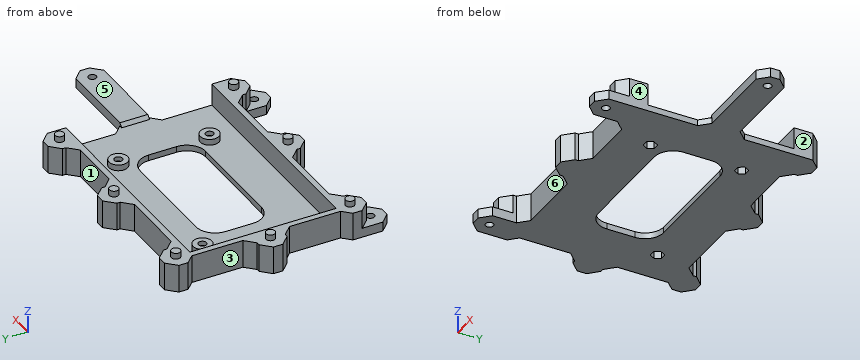
from build123d import *

# Parameters (mm, degrees)
F0_W          = 121.6
F0_H          = 78.3
F0_R          = 2.125
F1_DEPTH      = 3.2
F2_R          = 5
F2_R_2        = 2.125
F3_DEPTH      = 3.2
F5_DEPTH      = 4
F7_DEPTH      = 15
F8_R          = 2.425
F9_DEPTH      = 3.2
F11_W         = 15
F11_H         = 17.8
F11_R         = 2.125
F12_DEPTH     = 5
F13_T1_DEPTH  = 3.2
F13_T3_DEPTH  = 15
F13_T5_DEPTH  = 30.7168298797
F13_T7_DEPTH  = 22.8584149398
F13_T9_DEPTH  = 40.7168298797
F13_T14_DEPTH = 14.6584149398
F13_T19_DEPTH = 14.6584149398
F13_T24_DEPTH = 40.7168298797
F13_T29_DEPTH = 40.7168298797
F13_T34_DEPTH = 40.7168298797


# Not quite as in the source:
# - a fillet or chamfer that OpenCascade refuses, or shapes differently, is made with other operations: its cross-section is extruded or revolved along the edge and cut away or added
# - two fillets or chamfers of one size are made in one step
# - a feature of the source that left no trace in its solid (it failed there, or was rolled back) is left out
# - a feature names something its author has since deleted; it is built from what else it names


with BuildPart() as f1:
    # F0 (on Top) → F1 (new body)
    with BuildSketch(Plane.XY):
        Rectangle(F0_W, F0_H)
        with Locations((35.5, -24.05)):
            Circle(F0_R, mode=Mode.SUBTRACT)
        with BuildLine():
            ThreePointArc((37.5, -7.5), (34.5710678119, -14.5710678119), (27.5, -17.5))
            Line((27.5, -17.5), (-27.5, -17.5))
            ThreePointArc((-27.5, -17.5), (-34.5710678119, -14.5710678119), (-37.5, -7.5))
            Line((-37.5, -7.5), (-37.5, 7.5))
            ThreePointArc((-37.5, 7.5), (-34.5710678119, 14.5710678119), (-27.5, 17.5))
            Line((-27.5, 17.5), (27.5, 17.5))
            ThreePointArc((27.5, 17.5), (34.5710678119, 14.5710678119), (37.5, 7.5))
            Line((37.5, 7.5), (37.5, -7.5))
        make_face(mode=Mode.SUBTRACT)
        with Locations((-45.72, 24.15)):
            Circle(F0_R, mode=Mode.SUBTRACT)
        with Locations((36.8, 24.15)):
            Circle(F0_R, mode=Mode.SUBTRACT)
    extrude(amount=F1_DEPTH)

    # F2 (on face) → F3 (join)
    with BuildSketch(Plane.XY.offset(3.2)):
        with Locations((-45.72, 24.15)):
            Circle(F2_R)
        with Locations((-45.72, 24.15)):
            Circle(F2_R_2, mode=Mode.SUBTRACT)
        with Locations((36.8, 24.15)):
            Circle(F2_R)
        with Locations((36.8, 24.15)):
            Circle(F2_R_2, mode=Mode.SUBTRACT)
        with Locations((35.5, -24.05)):
            Circle(F2_R)
        with Locations((35.5, -24.05)):
            Circle(F2_R_2, mode=Mode.SUBTRACT)
    extrude(amount=F3_DEPTH)

    # F4 (on face) → F5 (cut)
    with BuildSketch(Plane(origin=(0, 0, 0), x_dir=(1, 0, 0), z_dir=(0, 0, -1))):
        Polygon((-44.0312504626, -21.225), (-47.4087495374, -21.225), (-49.0974990748, -24.15), (-47.4087495374, -27.075), (-44.0312504626, -27.075), (-42.3425009252, -24.15), align=None)
        Polygon((38.4887495374, -21.225), (35.1112504626, -21.225), (33.4225009252, -24.15), (35.1112504626, -27.075), (38.4887495374, -27.075), (40.1774990748, -24.15), align=None)
        Polygon((33.8112504626, 21.125), (37.1887495374, 21.125), (38.8774990748, 24.05), (37.1887495374, 26.975), (33.8112504626, 26.975), (32.1225009252, 24.05), align=None)
    extrude(amount=-F5_DEPTH, mode=Mode.SUBTRACT)

    # F6 (on Top) → F7 (join)
    with BuildSketch(Plane.XY):
        Polygon((-60.8, 39.15), (60.8, 39.15), (60.8, 54.15), (45.8, 54.15), (45.8, 42.35), (7.5, 42.35), (7.5, 54.15), (-7.5, 54.15), (-7.5, 42.35), (-53.3, 42.35), (-53.3, 54.15), (-68.3, 54.15), (-68.3, 39.15), (-64, 39.15), (-64, 7.5), (-75.8, 7.5), (-75.8, -7.5), (-64, -7.5), (-64, -39.15), (-68.3, -39.15), (-68.3, -54.15), (-53.3, -54.15), (-53.3, -42.35), (-7.5, -42.35), (-7.5, -54.15), (7.5, -54.15), (7.5, -42.35), (45.8, -42.35), (45.8, -54.15), (60.8, -54.15), (60.8, -39.15), (-60.8, -39.15), align=None)
    extrude(amount=F7_DEPTH)

    # F8 (on face) → F9 (join)
    with BuildSketch(Plane.XY.offset(15)):
        with Locations((53.3, 46.65)):
            Circle(F8_R)
        with Locations((0, 46.65)):
            Circle(F8_R)
        with Locations((-60.8, 46.65)):
            Circle(F8_R)
        with Locations((-68.3, 0)):
            Circle(F8_R)
        with Locations((-60.8, -46.65)):
            Circle(F8_R)
        with Locations((0, -46.65)):
            Circle(F8_R)
        with Locations((53.3, -46.65)):
            Circle(F8_R)
    extrude(amount=F9_DEPTH)

    # F11 (on Top) → F12 (join)
    with BuildSketch(Plane.XY):
        with Locations((53.3, -56.25)):
            Rectangle(F11_W, F11_H)
        with Locations((53.3, -57.65)):
            Circle(F11_R, mode=Mode.SUBTRACT)
        with Locations((-60.8, -56.25)):
            Rectangle(F11_W, F11_H)
        with Locations((-60.8, -57.65)):
            Circle(F11_R, mode=Mode.SUBTRACT)
        Polygon((60.8, -7.5), (64, -7.5), (114, -7.5), (114, 7.5), (64, 7.5), (60.8, 7.5), align=None)
        with Locations((106.5, 0)):
            Circle(F11_R, mode=Mode.SUBTRACT)
    extrude(amount=F12_DEPTH)

    # F13: chamfer of 5 on 37 edges, made by hand

    # F13_s2 → F13_t1 (join)
    with BuildSketch(Plane.XY):
        Polygon((65.8, 7.5), (60.8, 12.5), (60.8, 7.5), align=None)
        Polygon((60.8, -12.5), (65.8, -7.5), (60.8, -7.5), align=None)
    extrude(amount=F13_T1_DEPTH)

    # F13_s4 → F13_t3 (join)
    with BuildSketch(Plane.XY):
        Polygon((45.8, 47.35), (40.8, 42.35), (45.8, 42.35), align=None)
        Polygon((12.5, 42.35), (7.5, 47.35), (7.5, 42.35), align=None)
        Polygon((-7.5, 47.35), (-12.5, 42.35), (-7.5, 42.35), align=None)
        Polygon((-48.3, 42.35), (-53.3, 47.35), (-53.3, 42.35), align=None)
        Polygon((-64, 12.5), (-69, 7.5), (-64, 7.5), align=None)
        Polygon((-69, -7.5), (-64, -12.5), (-64, -7.5), align=None)
        Polygon((-53.3, -47.35), (-48.3, -42.35), (-53.3, -42.35), align=None)
        Polygon((-12.5, -42.35), (-7.5, -47.35), (-7.5, -42.35), align=None)
        Polygon((7.5, -47.35), (12.5, -42.35), (7.5, -42.35), align=None)
        Polygon((40.8, -42.35), (45.8, -47.35), (45.8, -42.35), align=None)
    extrude(amount=F13_T3_DEPTH)

    # F13_s6 → F13_t5 (cut)
    with BuildSketch(Plane.XY.offset(-12.8584149398)):
        Polygon((-68.3, -60.15), (-63.3, -65.15), (-68.3, -65.15), align=None)
        Polygon((-58.3, -65.15), (-53.3, -60.15), (-53.3, -65.15), align=None)
        Polygon((50.8, -65.15), (45.8, -60.15), (45.8, -65.15), align=None)
        Polygon((60.8, -60.15), (55.8, -65.15), (60.8, -65.15), align=None)
        Polygon((114, 2.5), (109, 7.5), (114, 7.5), align=None)
        Polygon((109, -7.5), (114, -2.5), (114, -7.5), align=None)
    extrude(amount=F13_T5_DEPTH, mode=Mode.SUBTRACT)

    # F13_s8 → F13_t7 (cut)
    with BuildSketch(Plane.XY.offset(5)):
        Polygon((60.8, -49.15), (55.8, -54.15), (60.8, -54.15), align=None)
        Polygon((-68.3, -49.15), (-63.3, -54.15), (-68.3, -54.15), align=None)
        Polygon((-53.3, -49.15), (-58.3, -54.15), (-53.3, -54.15), align=None)
        Polygon((50.8, -54.15), (45.8, -49.15), (45.8, -54.15), align=None)
    extrude(amount=F13_T7_DEPTH, mode=Mode.SUBTRACT)

    # F13_s10 → F13_t9 (cut)
    with BuildSketch(Plane.XY.offset(-12.8584149398)):
        Polygon((60.8, 49.15), (55.8, 54.15), (60.8, 54.15), align=None)
        Polygon((50.8, 54.15), (45.8, 49.15), (45.8, 54.15), align=None)
        Polygon((7.5, 49.15), (2.5, 54.15), (7.5, 54.15), align=None)
        Polygon((-2.5, 54.15), (-7.5, 49.15), (-7.5, 54.15), align=None)
        Polygon((-53.3, 49.15), (-58.3, 54.15), (-53.3, 54.15), align=None)
        Polygon((-63.3, 54.15), (-68.3, 49.15), (-68.3, 54.15), align=None)
        Polygon((-70.8, 7.5), (-75.8, 2.5), (-75.8, 7.5), align=None)
        Polygon((-75.8, -2.5), (-70.8, -7.5), (-75.8, -7.5), align=None)
        Polygon((-7.5, -49.15), (-2.5, -54.15), (-7.5, -54.15), align=None)
        Polygon((2.5, -54.15), (7.5, -49.15), (7.5, -54.15), align=None)
    extrude(amount=F13_T9_DEPTH, mode=Mode.SUBTRACT)


with BuildPart() as f13_tool12:
    # F13_s13 → F13_t14 (new body)
    with BuildSketch(Plane.XY.offset(3.2)):
        Polygon((65.8, 7.5), (60.8, 2.5), (60.8, 7.5), align=None)
    extrude(amount=F13_T14_DEPTH)

    split(bisect_by=Plane(origin=(30.4, 0, -30.4), x_dir=(0, 1, 0), z_dir=(-0.7071067812, 0, 0.7071067812)), keep=Keep.TOP)


with BuildPart() as f1_1:
    add(f1.part)

    # F13_t11: cut F13_tool12
    add(f13_tool12.part, mode=Mode.SUBTRACT)


with BuildPart() as f13_tool17:
    # F13_s18 → F13_t19 (new body)
    with BuildSketch(Plane.XY.offset(3.2)):
        Polygon((65.8, -7.5), (60.8, -2.5), (60.8, -7.5), align=None)
    extrude(amount=F13_T19_DEPTH)

    split(bisect_by=Plane(origin=(30.4, 0, -30.4), x_dir=(0, 1, 0), z_dir=(-0.7071067812, 0, 0.7071067812)), keep=Keep.TOP)


with BuildPart() as f1_2:
    add(f1_1.part)

    # F13_t16: cut F13_tool17
    add(f13_tool17.part, mode=Mode.SUBTRACT)


with BuildPart() as f13_tool22:
    # F13_s23 → F13_t24 (new body)
    with BuildSketch(Plane.XZ.offset(-20.3584149398)):
        Polygon((60.8, 0), (65.8, 5), (60.8, 5), align=None)
    extrude(amount=F13_T24_DEPTH)

    split(bisect_by=Plane.XY.offset(3.2), keep=Keep.TOP)


with BuildPart() as f1_3:
    add(f1_2.part)

    # F13_t21: cut F13_tool22
    add(f13_tool22.part, mode=Mode.SUBTRACT)


with BuildPart() as f13_tool27:
    # F13_s28 → F13_t29 (new body)
    with BuildSketch(Plane.XY.offset(-12.8584149398)):
        Polygon((-68.3, 44.15), (-63.3, 39.15), (-68.3, 39.15), align=None)
    extrude(amount=F13_T29_DEPTH)

    split(bisect_by=Plane.YZ.offset(-64), keep=Keep.BOTTOM)


with BuildPart() as f1_4:
    add(f1_3.part)

    # F13_t26: cut F13_tool27
    add(f13_tool27.part, mode=Mode.SUBTRACT)


with BuildPart() as f13_tool32:
    # F13_s33 → F13_t34 (new body)
    with BuildSketch(Plane.XY.offset(-12.8584149398)):
        Polygon((-63.3, -39.15), (-68.3, -44.15), (-68.3, -39.15), align=None)
    extrude(amount=F13_T34_DEPTH)

    split(bisect_by=Plane.YZ.offset(-64), keep=Keep.BOTTOM)


with BuildPart() as f1_5:
    add(f1_4.part)

    # F13_t31: cut F13_tool32
    add(f13_tool32.part, mode=Mode.SUBTRACT)


solid = f1_5.part
Geometry check sheet. Reference: the model listing, model coordinates, mm. Face numbers are marked on the shaded views. A direction names the side the tool comes from. Round coordinates to 2 decimals unless told otherwise and drop trailing zeros. Loops run counter-clockwise (first coordinate to the right, second up) from the corner with the lowest first, then second, coordinate; pieces in that order, holes last.
Item 1: Cross-section at C-C on y = -31.5. Record the boundary of the cut face in (x, z).
Item 2: Gauge pin test, flat ends, axial feed: pin 1 (2 mm diameter, centred on y = -48, z = 6, fed in from +X); pin 2 (2 mm diameter, centred on y = -25.5, z = 14, fed in from +X); pin 3 (8 mm diameter, centred on x = 33.5, y = -24.5, fed in from +Z). Record the tip position at first contact, or that the pin passes through.
Item 3: Thickness scan on line 1 (Y direction, x = 53.3, z = 3.45) (3 decimals); line 2 (Y direction, x = -60.8, z = 2.65) (3 decimals); line 3 (Y direction, x = -45.72, z = 5.25) (3 decimals). Record the ranges inside material, lowest first.
Item 4: Cross-section at A-A on x = 106.5. Record the boundary of the cut face in (y, z) (3 decimals).
Item 5: Access from +Z, -Z, +X, -X, +Y, -Y to the whole of each face (thin tool, end or side, straight path). Record for the marked faces 4, 5 and 6.
Item 6: Cross-section at D-D on x = -32.5. Record the boundary of the cut face in (y, z).
Item 7: Cross-section at B-B on y = 0. Record the boundary of the cut face in (x, z) (3 decimals).
Item 8: Mould release check, pull along X, two halves, no side actions. Record for the marked faces 1, 2 and 3: pulls with the +X half, pulls with the -X half, needs draft (parallel to the pull), parting line crosses it, or undercut.
Answer sheet:
1. outline: (-64, 0) - (60.8, 0) - (60.8, 3.2) - (-60.8, 3.2) - (-60.8, 15) - (-64, 15) - close
2. pin 1: stops at x = 60.8
2. pin 2: stops at x = -60.8
2. pin 3: stops at z = 6.4
3. line 1: y = -65.15 to -59.775, -55.525 to -39.15, 39.15 to 54.15
3. line 2: y = -65.15 to -59.775, -55.525 to 54.15
3. line 3: y = -42.35 to -39.15, 19.15 to 22.025, 26.275 to 29.15, 39.15 to 42.35
4. outline: (-7.5, 0) - (-2.125, 0) - (-2.125, 5) - (-7.5, 5) - close; (2.125, 0) - (7.5, 0) - (7.5, 5) - (2.125, 5) - close
5. face 4: +Z, -Z, +X, -Y
5. face 5: +Z, +X, +Y, -Y
5. face 6: +Z, -Z, -Y
6. outline: (-42.35, 0) - (-16.16, 0) - (-16.16, 3.2) - (-39.15, 3.2) - (-39.15, 15) - (-42.35, 15) - close; (16.16, 0) - (42.35, 0) - (42.35, 15) - (39.15, 15) - (39.15, 3.2) - (16.16, 3.2) - close
7. outline: (-75.8, 0) - (-37.5, 0) - (-37.5, 3.2) - (-60.8, 3.2) - (-60.8, 15) - (-65.875, 15) - (-65.875, 18.2) - (-70.725, 18.2) - (-70.725, 15) - (-75.8, 15) - close; (37.5, 0) - (104.375, 0) - (104.375, 5) - (65.8, 5) - (64, 3.2) - (37.5, 3.2) - close; (108.625, 0) - (114, 0) - (114, 5) - (108.625, 5) - close
8. face 1: undercut
8. face 2: pulls with the +X half
8. face 3: pulls with the -X half
